from build123d import *

# Parameters (mm, degrees)
EXTRUDE1_DEPTH = 2.794
CHAMFER1_SIZE  = 0.508
CHAMFER2_SIZE  = 0.29329394
CHAMFER2_SIZE2 = 0.253999961


with BuildPart() as part:
    # Sketch1 → Revolve1 (revolve)
    with BuildSketch(Plane.XY, mode=Mode.PRIVATE) as revolve1_sk:
        Polygon((0, 0), (0, 17.4752), (-3.9116, 17.4752), (-3.9116, 12.7), (-2.3876, 12.7), (-2.3876, 0), align=None)
    revolve(revolve1_sk.sketch.rotate(Axis((0, 0, 0), (0, 1, 0)), 270), axis=Axis((0, 0, 0), (0, 1, 0)))

    # Sketch2 → Extrude1 (cut)
    with BuildSketch(Plane(origin=(0, 17.4752, 0), x_dir=(1, 0, 0), z_dir=(0, 1, 0))):
        Polygon((2.2913594, 0), (1.1456797, 1.98437545), (-1.1456797, 1.98437545), (-2.2913594, 0), (-1.1456797, -1.98437545), (1.1456797, -1.98437545), align=None)
    extrude(amount=-EXTRUDE1_DEPTH, mode=Mode.SUBTRACT)

    # Chamfer1
    chamfer1_edges = [part.edges().sort_by_distance(p)[0] for p in [
        (0, 0, 2.3876),
        (0, 17.4752, 3.9116),
    ]]
    chamfer(chamfer1_edges, length=CHAMFER1_SIZE)

    # Chamfer2
    chamfer2_edges = [part.edges().sort_by_distance(p)[0] for p in [
        (1.71851955, 17.4752, 0.992187725),
        (1.71851955, 17.4752, -0.992187725),
        (0, 17.4752, -1.98437545),
        (-1.71851955, 17.4752, -0.992187725),
        (-1.71851955, 17.4752, 0.992187725),
        (0, 17.4752, 1.98437545),
    ]]
    chamfer2_side = [part.faces().sort_by_distance(p)[0] for p in [
        (0, 17.4752, 3.307331654),
    ]]
    chamfer(chamfer2_edges, length=CHAMFER2_SIZE, length2=CHAMFER2_SIZE2, reference=chamfer2_side[0])


solid = part.part
Part model, mm, in its own coordinate system. A direction names the side the tool comes from. Give positions to 0.01 mm unless a question says otherwise; leave off trailing zeros. Order: outer loops, then holes, each group sorted by start corner. A loop starts at its lowest first (then second) coordinate and runs counter-clockwise, first axis right, second up. Notation, with made-up numbers: (65.5, 6) -> (86.5, 6) arc R24 ccw to (86.5, 35) -> close; hole circle Ø2 at (11, -14.75). An arc over 180 degrees is marked (long way). Use one line per item in the form item = value.
(1) Saw through at D-D (y = 13.75). Write the cut outline in (x, z), then the cut area to 3 significant figures.
Solution:
outline = circle Ø7.82 at (0, 0)
area = 48.1 mm²
(2) Tool access for faces 4 (the face through (2.33, 6.52, 0.52)), 5 (the face through (-1.727, 15.969, 0.978)), 6 (the face through (0, 0, 0)): list every direction of +Z, -Z, +X, -X, +Y, -Y with a clear straight run to the whole face (end or side of a thin tool).
Solution:
face_4 = -Y
face_5 = +Y
face_6 = +Z, -Z, +X, -X, -Y
(3) Saw through at B-B (x = 0). Write the cut outline in (y, z).
Solution:
outline = (0, -1.88) -> (0.51, -2.39) -> (12.7, -2.39) -> (12.7, -3.91) -> (16.97, -3.91) -> (17.48, -3.4) -> (17.48, -2.28) -> (17.22, -1.98) -> (14.68, -1.98) -> (14.68, 1.98) -> (17.22, 1.98) -> (17.48, 2.28) -> (17.48, 3.4) -> (16.97, 3.91) -> (12.7, 3.91) -> (12.7, 2.39) -> (0.51, 2.39) -> (0, 1.88) -> close
(4) Saw through at C-C (y = 9.25). Write the cut outline in (x, z), then the cut area to 3 significant figures.
Solution:
outline = circle Ø4.78 at (0, 0)
area = 17.9 mm²
(5) Saw through at A-A (y = 15.5). Write the cut outline in (x, z).
Solution:
outline = circle Ø7.82 at (0, 0); hole (-2.29, 0) -> (-1.15, -1.98) -> (1.15, -1.98) -> (2.29, 0) -> (1.15, 1.98) -> (-1.15, 1.98) -> close
(6) Drill centre lines: line 1 (Z direction, x = -0.5, y = 15.5); line 2 (Y direction, x = -0.25, z = -2.5); line 3 (Y direction, x = -1, z = -1.5). Where is each one in solid material? Low to high. Write a range as from..to.
Solution:
line_1 = -3.88..-1.98, 1.98..3.88
line_2 = 12.7..17.48
line_3 = 0..14.68
(7) Pull direction Z, two halves, no side cores. Call faces 1 (the face through (-2, 12.7, -2)), 2 (the face through (-1.175, 14.804, -3.731)), 3 (the face through (1.853, 17.346, -1.049)): +Z half, -Z half, draft (parallel to the pull), parting line (faces both ways), or undercut.
Solution:
face_1 = draft
face_2 = parting line
face_3 = undercut
(8) Flat gauge pins, fed straight in: P1, Ø2, axis at y = 8.5, z = -1, coming from the +X side; P2, Ø3, axis at x = 0.5, z = -0.5, coming from the +Y side; P3, Ø4, axis at y = 5, z = 0.5, coming from the -X side. Where does each tip first touch, or does it go through?
Solution:
P1 = 2.39
P2 = 17.39
P3 = -2.39
